from build123d import *

# Parameters (mm, degrees)
F0_W     = 59.68371
F0_H     = 44.711508
F0_W_2   = 50
F0_H_2   = 25.664362
F0_W_3   = 39.789142
F0_H_3   = 19.586922
F0_W_4   = 3
F0_H_4   = 5.5
F1_DEPTH = 2


with BuildPart() as f1:
    # F0 (on Top) → F1 (new body)
    with BuildSketch(Plane.XY):
        with Locations((0.514649, -4.717808)):
            Rectangle(F0_W, F0_H)
        Rectangle(F0_W_2, F0_H_2, mode=Mode.SUBTRACT)
        Rectangle(F0_W_2, F0_H_2)
        with Locations((-0.203197, 0.358383)):
            Rectangle(F0_W_3, F0_H_3, mode=Mode.SUBTRACT)
        with Locations((-22.652147, 7.080561)):
            Rectangle(F0_W_4, F0_H_4, mode=Mode.SUBTRACT)
        with Locations((22.410813, 7.41029)):
            Rectangle(F0_W_4, F0_H_4, mode=Mode.SUBTRACT)
    extrude(amount=-F1_DEPTH)


solid = f1.part
Build history of the part. All positions in model axes, mm. A direction names the side the tool comes from. Round coordinates to 2 decimals unless told otherwise and drop trailing zeros. Loops run counter-clockwise (first coordinate to the right, second up) from the corner with the lowest first, then second, coordinate; pieces in that order, holes last. Notation, with made-up numbers: (19, -4) -> (48, -4) arc R9 ccw to (48, 1) -> close; hole circle Ø7 at (-34.5, 47). An arc over 180 degrees is marked (long way). Use CSV: the item, a comma, the result in double quotes. Start each with the question number.
Q1. Saw through at D-D on y = -3. Give the cut face in (x, z).
Q2. Saw through at B-B on y = 9. Give the cut face in (x, z).
Q3. Drill centre lines: L1, parallel to Y at x = 18, z = -0.8; L2, parallel to X at y = -9, z = -0.2; L3, parallel to Y at x = -23.5, z = -1. Where is each one in solid material? Low to high.
Q4. Saw through at C-C on z = -1.4. Give the cut face in (x, y), and give its area (3 significant figures).
Q5. Saw through at A-A on x = 11. Give the cut face in (y, z), and give its area (3 significant figures).
Q6. Which spindle directions (+Z, -Z, +X, -X, +Y, -Y) get a long thin tool onto all of the face, cutting with end or side? Do faces 1 (the face through (0, 10.152, -1)), 2 (the face through (0, -14, -2)). Say none if no direction does.
Q7. Mould opens along Y. For faces 3 (the face through (23.911, 7, -1)), 4 (the face through (30.357, -5, -1)), 5 (the face through (0, 17.638, -1)) say: +Y half, -Y half, draft (parallel to the pull), parting line (faces both ways), or undercut.
Solutions:
1,outline,"(-29.33, -2) -> (-20.1, -2) -> (-20.1, 0) -> (-29.33, 0) -> close; (19.69, -2) -> (30.36, -2) -> (30.36, 0) -> (19.69, 0) -> close"
2,outline,"(-29.33, -2) -> (-24.15, -2) -> (-24.15, 0) -> (-29.33, 0) -> close; (-21.15, -2) -> (-20.1, -2) -> (-20.1, 0) -> (-21.15, 0) -> close; (19.69, -2) -> (20.91, -2) -> (20.91, 0) -> (19.69, 0) -> close; (23.91, -2) -> (30.36, -2) -> (30.36, 0) -> (23.91, 0) -> close"
3,L1,"y = -27.07 to -9.44, 10.15 to 17.64"
3,L2,"x = -29.33 to -20.1, 19.69 to 30.36"
3,L3,"y = -27.07 to 4.33, 9.83 to 17.64"
4,outline,"(-29.33, -27.07) -> (30.36, -27.07) -> (30.36, 17.64) -> (-29.33, 17.64) -> close; hole (-24.15, 4.33) -> (-21.15, 4.33) -> (-21.15, 9.83) -> (-24.15, 9.83) -> close; hole (-20.1, -9.44) -> (19.69, -9.44) -> (19.69, 10.15) -> (-20.1, 10.15) -> close; hole (20.91, 4.66) -> (23.91, 4.66) -> (23.91, 10.16) -> (20.91, 10.16) -> close"
4,area,"1,860 mm^2"
5,outline,"(-27.07, -2) -> (-9.44, -2) -> (-9.44, 0) -> (-27.07, 0) -> close; (10.15, -2) -> (17.64, -2) -> (17.64, 0) -> (10.15, 0) -> close"
5,area,"50.2 mm^2"
6,face 1,"+Z, -Z"
6,face 2,"-Z, +X, -X, +Y, -Y"
7,face 3,"undercut"
7,face 4,"draft"
7,face 5,"+Y half"
